```python
from build123d import *

# Parameters (mm, degrees)
F1_DEPTH     = 27.94
F2_R         = 12.7
F3_DEPTH     = 30.48
F4_R         = 8.0083112146
F5_DEPTH     = 50.8
F6_W         = 13.97
F6_H         = 30.48
F7_DEPTH     = 19.05
F8_T1_DEPTH  = 21.823361814
F8_T3_DEPTH  = 21.823361814
F8_T5_DEPTH  = 20.4806552744
F8_T7_DEPTH  = 49.996723628
F8_T9_DEPTH  = 65.0760683536
F8_T14_DEPTH = 5.08
F8_T20_DEPTH = 5.08
F9_R         = 2.54
F10_DEPTH    = 20.321
F12_R        = 4.445
F13_DEPTH    = 25.4


# Not quite as in the source:
# - a fillet or chamfer that OpenCascade refuses, or shapes differently, is made with other operations: its cross-section is extruded or revolved along the edge and cut away or added


with BuildPart() as f1:
    # F0 (on Right) → F1 (new body, symmetric)
    with BuildSketch(Plane.YZ):
        Polygon((-16.0675346851, 10.16), (-16.0675346851, 0), (19.4924653149, 0), (19.4924653149, 35.56), (14.4124653149, 35.56), align=None)
    extrude(amount=F1_DEPTH, both=True)

    # F2 (on face) → F3 (cut)
    with BuildSketch(Plane.XY.offset(35.56)):
        Circle(F2_R)
    extrude(amount=-F3_DEPTH, mode=Mode.SUBTRACT)

    # F4 (on face) → F5 (cut)
    with BuildSketch(Plane.XY.offset(5.08)):
        Circle(F4_R)
    extrude(amount=-F5_DEPTH, mode=Mode.SUBTRACT)

    # F6 (on face) → F7 (cut)
    with BuildSketch(Plane.XZ.offset(16.0675346851)):
        Rectangle(F6_W, F6_H)
    extrude(amount=-F7_DEPTH, mode=Mode.SUBTRACT)

    # F8: fillet of radius 5.08 on 7 edges, made by hand

    # F8_s2 → F8_t1 (cut)
    with BuildSketch(Plane.YZ.offset(-22.86)):
        with BuildLine():
            ThreePointArc((-16.0675346851, 7.7806552744), (-15.587928945, 9.9353646873), (-14.2396714354, 11.6832193748))
            Line((-14.2396714354, 11.6832193748), (-16.0675346851, 10.16))
            Line((-16.0675346851, 10.16), (-16.0675346851, 7.7806552744))
        make_face()
    extrude(amount=F8_T1_DEPTH, mode=Mode.SUBTRACT)

    # F8_s4 → F8_t3 (cut)
    with BuildSketch(Plane.YZ.offset(1.036638186)):
        with BuildLine():
            ThreePointArc((-16.0675346851, 7.7806552744), (-15.587928945, 9.9353646873), (-14.2396714354, 11.6832193748))
            Line((-14.2396714354, 11.6832193748), (-16.0675346851, 10.16))
            Line((-16.0675346851, 10.16), (-16.0675346851, 7.7806552744))
        make_face()
    extrude(amount=F8_T3_DEPTH, mode=Mode.SUBTRACT)

    # F8_s6 → F8_t5 (cut)
    with BuildSketch(Plane.XY.offset(-12.7)):
        with BuildLine():
            ThreePointArc((27.94, -10.9875346851), (26.4521024484, -14.5796371336), (22.86, -16.0675346851))
            Line((22.86, -16.0675346851), (27.94, -16.0675346851))
            Line((27.94, -16.0675346851), (27.94, -10.9875346851))
        make_face()
        with BuildLine():
            ThreePointArc((-22.86, -16.0675346851), (-26.4521024484, -14.5796371336), (-27.94, -10.9875346851))
            Line((-27.94, -10.9875346851), (-27.94, -16.0675346851))
            Line((-27.94, -16.0675346851), (-22.86, -16.0675346851))
        make_face()
    extrude(amount=F8_T5_DEPTH, mode=Mode.SUBTRACT)

    # F8_s8 → F8_t7 (cut)
    with BuildSketch(Plane(origin=(0, 35.7506520761, 29.7922100634), x_dir=(1, 0, 0), z_dir=(0, -0.7682212796, -0.6401843997))):
        with BuildLine():
            ThreePointArc((27.94, 13.0113132472), (26.4521024484, 16.6034156956), (22.86, 18.0913132472))
            Line((22.86, 18.0913132472), (27.94, 18.0913132472))
            Line((27.94, 18.0913132472), (27.94, 13.0113132472))
        make_face()
        with BuildLine():
            ThreePointArc((-27.94, 13.0113132472), (-26.4521024484, 16.6034156956), (-22.86, 18.0913132472))
            Line((-22.86, 18.0913132472), (-27.94, 18.0913132472))
            Line((-27.94, 18.0913132472), (-27.94, 13.0113132472))
        make_face()
    extrude(amount=F8_T7_DEPTH, mode=Mode.SUBTRACT)

    # F8_s10 → F8_t9 (cut)
    with BuildSketch(Plane.YZ.offset(-32.5380341768)):
        with BuildLine():
            ThreePointArc((16.2516789856, 35.56), (14.5223186457, 35.2565796146), (12.9995422353, 34.3825641004))
            Line((12.9995422353, 34.3825641004), (14.4124653149, 35.56))
            Line((14.4124653149, 35.56), (16.2516789856, 35.56))
        make_face()
    extrude(amount=F8_T9_DEPTH, mode=Mode.SUBTRACT)


with BuildPart() as f8_tool12:
    # F8_s13 → F8_t14 (new body)
    with BuildSketch(Plane.YZ.offset(-22.86)):
        Polygon((-10.9875346851, 7.7806552744), (-14.2396714354, 11.6832193748), (-16.0675346851, 10.16), (-16.0675346851, 7.7806552744), align=None)
    extrude(amount=-F8_T14_DEPTH)

    # F8_s15 → F8_t16 (revolve, cut)
    with BuildSketch(Plane(origin=(-22.86, -10.9875346851, 7.7806552744), x_dir=(0, 0.9055894212, -0.4241553962), z_dir=(0, 0.4241553962, 0.9055894212))):
        with BuildLine():
            ThreePointArc((0, -5.08), (5.08, 0), (0, 5.08))
            Line((0, 5.08), (0, -5.08))
        make_face()
    revolve(axis=Axis((-22.86, -10.9875346851, 7.7806552744), (-1, 0, 0)), mode=Mode.SUBTRACT)


with BuildPart() as f1_1:
    add(f1.part)

    # F8_t11: cut F8_tool12
    add(f8_tool12.part, mode=Mode.SUBTRACT)


with BuildPart() as f8_tool18:
    # F8_s19 → F8_t20 (new body)
    with BuildSketch(Plane.YZ.offset(22.86)):
        Polygon((-10.9875346851, 7.7806552744), (-16.0675346851, 7.7806552744), (-16.0675346851, 10.16), (-14.2396714354, 11.6832193748), align=None)
    extrude(amount=F8_T20_DEPTH)

    # F8_s21 → F8_t22 (revolve, cut)
    with BuildSketch(Plane(origin=(22.86, -10.9875346851, 7.7806552744), x_dir=(0, 0.9055894212, -0.4241553962), z_dir=(0, -0.4241553962, -0.9055894212))):
        with BuildLine():
            ThreePointArc((0, -5.08), (5.08, 0), (0, 5.08))
            Line((0, 5.08), (0, -5.08))
        make_face()
    revolve(axis=Axis((22.86, -10.9875346851, 7.7806552744), (1, 0, 0)), mode=Mode.SUBTRACT)


with BuildPart() as f1_2:
    add(f1_1.part)

    # F8_t17: cut F8_tool18
    add(f8_tool18.part, mode=Mode.SUBTRACT)

    # F9 (on face) → F10 (cut, through all)
    with BuildSketch(Plane(origin=(0, 19.4924653149, 0), x_dir=(-1, 0, 0), z_dir=(0, 1, 0))):
        with Locations((-17.78, 25.4)):
            Circle(F9_R)
        with Locations((17.78, 25.4)):
            Circle(F9_R)
    extrude(amount=-F10_DEPTH, mode=Mode.SUBTRACT)

    # F12 (on offset) → F13 (cut)
    with BuildSketch(Plane(origin=(0, 14.4124653149, 0), x_dir=(-1, 0, 0), z_dir=(0, 1, 0))):
        with Locations((-17.78, 25.4)):
            Circle(F12_R)
        with Locations((17.78, 25.4)):
            Circle(F12_R)
    extrude(amount=-F13_DEPTH, mode=Mode.SUBTRACT)


solid = f1_2.part
```
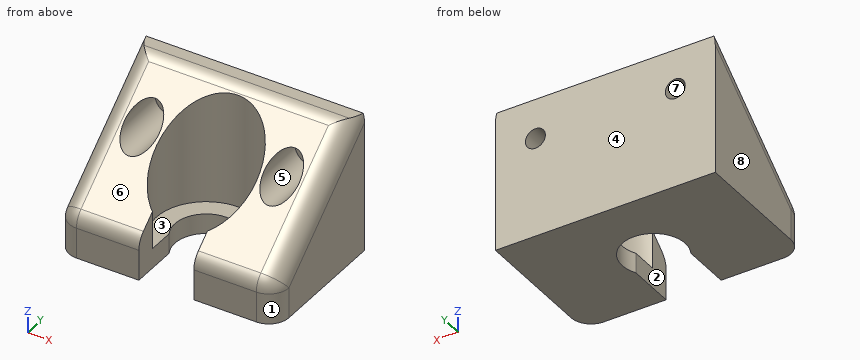
Can you work these out from the model? Positions are in its coordinate system, mm. Face numbers are marked on the shaded views. A direction names the side the tool comes from. Give positions to 0.01 mm unless a question says otherwise; leave off trailing zeros. Order: outer loops, then holes, each group sorted by start corner. A loop starts at its lowest first (then second) coordinate and runs counter-clockwise, first axis right, second up. Notation, with made-up numbers: (4, -26) - (47, -26) arc R9 ccw to (47, -10) - close; hole circle Ø5 at (34.25, -31). An arc over 180 degrees is marked (long way). Use a Markdown table: item, result. Add a question column.
Q1. If we section it at C-C on x = 0: Write out the boundary of the cut face in (y, z).
Q2. If we mould it in two halves opening along Z, with no side actions, what happens to the marked faces 6, 7 and 8? For each: released by +Z, released by -Z, zero draft, split by the parting line, or undercut.
Q3. If we section it at A-A on z = 3.5: Write out the boundary of the cut face in (x, y) (3 decimals), plus the area to 3 significant figures.
Q4. If we section it at D-D on z = 25.4: Count the separate pieces of the cut face and the enclosed holes in it, plus the area to 3 significant figures.
Q5. Please list where these lines run through material, in increasing order: line 1 along Z through (x, y) = (-17.78, 16.4); line 2 along X through (y, z) = (0, 3.85); line 3 along X through (y, z) = (6, 25).
Q6. If we section it at B-B on x = -17.5: Write out the boundary of the cut face in (y, z), plus the area to 3 significant figures.
Q7. I'm going to push flat-ended pins straight in: pin 1 (3 mm diameter, centred on x = 17.78, z = 25.4, fed in from +Y); pin 2 (11.5 mm diameter, centred on x = -17.78, z = 25.4, fed in from -Y); pin 3 (4 mm diameter, centred on x = 13.5, y = -0.5, fed in from +Z); pin 4 (2 mm diameter, centred on x = -5.5, y = 10, fed in from -Z). Where does each tip first touch, or does it pass through?
Q8. On a 3-axis mill with a long thin cutter (end or side, diameter ignored), from which of +Z, -Z, +X, -X, +Y, -Y can I reach the whole of each face in a straight line? I mean the marked faces 1, 2, 3, 4 and 5. Say none if no direction works.
Answers follow:
| question | item | result |
|---|---|---|
| 1 | outline | (8.01, 0) - (19.49, 0) - (19.49, 35.56) - (16.25, 35.56) arc R5.08 ccw to (13, 34.38) - (12.7, 34.13) - (12.7, 5.08) - (8.01, 5.08) - close |
| 2 | face 6 | released by +Z |
| 2 | face 7 | undercut |
| 2 | face 8 | zero draft |
| 3 | outline | (-27.94, -10.988) arc R5.08 ccw to (-22.86, -16.068) - (-6.985, -16.068) - (-6.985, -3.917) arc R8.008 cw (long way) to (6.985, -3.917) - (6.985, -16.068) - (22.86, -16.068) arc R5.08 ccw to (27.94, -10.988) - (27.94, 19.492) - (-27.94, 19.492) - close |
| 3 | area | 1,650 mm^2 |
| 4 | separate pieces | 3 |
| 4 | enclosed holes | 0 |
| 4 | area | 482 mm^2 |
| 5 | line 1 | z = 0 to 22.86, 27.94 to 35.56 |
| 5 | line 2 | x = -27.94 to -8.01, 8.01 to 27.94 |
| 5 | line 3 | x = -27.36 to -22.21, -13.35 to -11.19, 11.19 to 13.35, 22.21 to 27.36 |
| 6 | outline | (-16.07, 0) - (19.49, 0) - (19.49, 22.88) - (14.41, 22.88) - (14.41, 20.96) - (-3.1, 20.96) - (-14.24, 11.68) arc R5.08 ccw to (-16.07, 7.78) - close; (7.54, 29.84) - (14.41, 29.84) - (14.41, 27.92) - (19.49, 27.92) - (19.49, 35.56) - (16.25, 35.56) arc R5.08 ccw to (13, 34.38) - close |
| 6 | area | 742 mm^2 |
| 7 | pin 1 | passes through |
| 7 | pin 2 | stops at y = -4.68 |
| 7 | pin 3 | stops at z = 24.8 |
| 7 | pin 4 | stops at z = 0 |
| 8 | face 1 | +Z, -Z, +X, -Y |
| 8 | face 2 | +Z, -Z, -Y |
| 8 | face 3 | +Z |
| 8 | face 4 | +Z, -Z, +X, -X, +Y |
| 8 | face 5 | -Y |
